from build123d import *

# Parameters (mm, degrees)
BOSS_EXTRUDE2_DEPTH = 39
SKETCH5_R           = 3
BOSS_EXTRUDE3_DEPTH = 0.75
BOSS_EXTRUDE5_DEPTH = 10
SKETCH10_R          = 2.25
BOSS_EXTRUDE6_DEPTH = 0.5


with BuildPart() as part:
    # Sketch4 → Boss-Extrude2 (new body)
    with BuildSketch(Plane(origin=(0, 0, 0), x_dir=(1, 0, 0), z_dir=(0, 1, 0))):
        with BuildLine():
            Line((-0.32, 1.337245303), (-0.32, 0.32))
            Line((-0.32, 0.32), (-1.337245303, 0.32))
            ThreePointArc((-1.337245303, 0.32), (-1.375, 0), (-1.337245303, -0.32))
            Line((-1.337245303, -0.32), (-0.32, -0.32))
            Line((-0.32, -0.32), (-0.32, -1.337245303))
            ThreePointArc((-0.32, -1.337245303), (0, -1.375), (0.32, -1.337245303))
            Line((0.32, -1.337245303), (0.32, -0.32))
            Line((0.32, -0.32), (1.337245303, -0.32))
            ThreePointArc((1.337245303, -0.32), (1.375, 0), (1.337245303, 0.32))
            Line((1.337245303, 0.32), (0.32, 0.32))
            Line((0.32, 0.32), (0.32, 1.337245303))
            ThreePointArc((0.32, 1.337245303), (0, 1.375), (-0.32, 1.337245303))
        make_face()
    extrude(amount=BOSS_EXTRUDE2_DEPTH)

    # Sketch5 → Boss-Extrude3 (add)
    with BuildSketch(Plane(origin=(0, 39, 0), x_dir=(1, 0, 0), z_dir=(0, 1, 0))):
        with Locations(Location((0, 0, 0), (0, 0, 270))):
            Circle(SKETCH5_R)
    extrude(amount=BOSS_EXTRUDE3_DEPTH)

    # Sketch9 → Boss-Extrude5 (add)
    with BuildSketch(Plane(origin=(0, 39.75, 0), x_dir=(1, 0, 0), z_dir=(0, 1, 0))):
        with BuildLine():
            Line((-0.83040283, -2.358056645), (-0.873204905, -2.479599724))
            ThreePointArc((-0.873204905, -2.479599724), (-0.653770741, -2.546268921), (-0.429360987, -2.593559473))
            Line((-0.429360987, -2.593559473), (-0.408314906, -2.466430404))
            ThreePointArc((-0.408314906, -2.466430404), (-0.313333084, -2.480286753), (-0.217889357, -2.490486745))
            Line((-0.217889357, -2.490486745), (-0.229120191, -2.618855769))
            ThreePointArc((-0.229120191, -2.618855769), (0, -2.628859372), (0.229120191, -2.618855769))
            Line((0.229120191, -2.618855769), (0.217889357, -2.490486745))
            ThreePointArc((0.217889357, -2.490486745), (0.313333084, -2.480286753), (0.408314906, -2.466430404))
            Line((0.408314906, -2.466430404), (0.429360987, -2.593559473))
            ThreePointArc((0.429360987, -2.593559473), (0.653770741, -2.546268921), (0.873204905, -2.479599724))
            Line((0.873204905, -2.479599724), (0.83040283, -2.358056645))
            ThreePointArc((0.83040283, -2.358056645), (0.920311382, -2.324441215), (1.008863241, -2.28739917))
            Line((1.008863241, -2.28739917), (1.060863834, -2.405300298))
            ThreePointArc((1.060863834, -2.405300298), (1.266462661, -2.303687029), (1.462422943, -2.18454131))
            Line((1.462422943, -2.18454131), (1.390739039, -2.077461173))
            ThreePointArc((1.390739039, -2.077461173), (1.469463131, -2.022542486), (1.546020988, -1.964642233))
            Line((1.546020988, -1.964642233), (1.625708706, -2.065907259))
            ThreePointArc((1.625708706, -2.065907259), (1.799578075, -1.916356008), (1.959751569, -1.752220131))
            Line((1.959751569, -1.752220131), (1.863689999, -1.666331176))
            ThreePointArc((1.863689999, -1.666331176), (1.926283107, -1.593559974), (1.986036551, -1.518439599))
            Line((1.986036551, -1.518439599), (2.088404321, -1.596705669))
            ThreePointArc((2.088404321, -1.596705669), (2.21961938, -1.408613292), (2.333941796, -1.209800517))
            Line((2.333941796, -1.209800517), (2.219538463, -1.150499462))
            ThreePointArc((2.219538463, -1.150499462), (2.262067631, -1.064448229), (2.301262134, -0.976827821))
            Line((2.301262134, -0.976827821), (2.419877811, -1.027177189))
            ThreePointArc((2.419877811, -1.027177189), (2.500193836, -0.812362222), (2.561481877, -0.591364688))
            Line((2.561481877, -0.591364688), (2.435925162, -0.562377636))
            ThreePointArc((2.435925162, -0.562377636), (2.455718127, -0.468453286), (2.471890953, -0.373838359))
            Line((2.471890953, -0.373838359), (2.599301479, -0.393107389))
            ThreePointArc((2.599301479, -0.393107389), (2.623671919, -0.165067446), (2.628074631, 0.064228761))
            Line((2.628074631, 0.064228761), (2.499253724, 0.061080445))
            ThreePointArc((2.499253724, 0.061080445), (2.495066821, 0.156976299), (2.487201772, 0.252640743))
            Line((2.487201772, 0.252640743), (2.615401476, 0.265662794))
            ThreePointArc((2.615401476, 0.265662794), (2.582295045, 0.492599125), (2.52953579, 0.715786479))
            Line((2.52953579, 0.715786479), (2.405544984, 0.680700618))
            ThreePointArc((2.405544984, 0.680700618), (2.377641291, 0.772542486), (2.346232557, 0.863245497))
            Line((2.346232557, 0.863245497), (2.467166179, 0.907740407))
            ThreePointArc((2.467166179, 0.907740407), (2.378663077, 1.119313881), (2.272056913, 1.322368701))
            Line((2.272056913, 1.322368701), (2.160687005, 1.257549867))
            ThreePointArc((2.160687005, 1.257549867), (2.110819814, 1.339566987), (2.057840921, 1.419609363))
            Line((2.057840921, 1.419609363), (2.163909757, 1.492781351))
            ThreePointArc((2.163909757, 1.492781351), (2.02557096, 1.67569803), (1.871816344, 1.845861634))
            Line((1.871816344, 1.845861634), (1.780065115, 1.755382632))
            ThreePointArc((1.780065115, 1.755382632), (1.711367765, 1.822421569), (1.640147572, 1.886773951))
            Line((1.640147572, 1.886773951), (1.724686927, 1.984025353))
            ThreePointArc((1.724686927, 1.984025353), (1.545204769, 2.126791908), (1.35396267, 2.253372292))
            Line((1.35396267, 2.253372292), (1.287595187, 2.142918252))
            ThreePointArc((1.287595187, 2.142918252), (1.204384185, 2.1907667), (1.11939772, 2.235385592))
            Line((1.11939772, 2.235385592), (1.177095675, 2.350605746))
            ThreePointArc((1.177095675, 2.350605746), (0.96774768, 2.444251629), (0.751034542, 2.519295281))
            Line((0.751034542, 2.519295281), (0.714220919, 2.395806436))
            ThreePointArc((0.714220919, 2.395806436), (0.621724718, 2.421457903), (0.528311991, 2.443539736))
            Line((0.528311991, 2.443539736), (0.555543172, 2.569488934))
            ThreePointArc((0.555543172, 2.569488934), (0.329483446, 2.608130031), (0.100916152, 2.626921683))
            Line((0.100916152, 2.626921683), (0.095969523, 2.498157291))
            ThreePointArc((0.095969523, 2.498157291), (0, 2.5), (-0.095969523, 2.498157291))
            Line((-0.095969523, 2.498157291), (-0.100916152, 2.626921683))
            ThreePointArc((-0.100916152, 2.626921683), (-0.329483446, 2.608130031), (-0.555543172, 2.569488934))
            Line((-0.555543172, 2.569488934), (-0.528311991, 2.443539736))
            ThreePointArc((-0.528311991, 2.443539736), (-0.621724718, 2.421457903), (-0.714220919, 2.395806436))
            Line((-0.714220919, 2.395806436), (-0.751034542, 2.519295281))
            ThreePointArc((-0.751034542, 2.519295281), (-0.96774768, 2.444251629), (-1.177095675, 2.350605746))
            Line((-1.177095675, 2.350605746), (-1.11939772, 2.235385592))
            ThreePointArc((-1.11939772, 2.235385592), (-1.204384185, 2.1907667), (-1.287595187, 2.142918252))
            Line((-1.287595187, 2.142918252), (-1.35396267, 2.253372292))
            ThreePointArc((-1.35396267, 2.253372292), (-1.545204769, 2.126791908), (-1.724686927, 1.984025353))
            Line((-1.724686927, 1.984025353), (-1.640147572, 1.886773951))
            ThreePointArc((-1.640147572, 1.886773951), (-1.711367765, 1.822421569), (-1.780065115, 1.755382632))
            Line((-1.780065115, 1.755382632), (-1.871816344, 1.845861634))
            ThreePointArc((-1.871816344, 1.845861634), (-2.02557096, 1.67569803), (-2.163909757, 1.492781351))
            Line((-2.163909757, 1.492781351), (-2.057840921, 1.419609363))
            ThreePointArc((-2.057840921, 1.419609363), (-2.110819814, 1.339566987), (-2.160687005, 1.257549867))
            Line((-2.160687005, 1.257549867), (-2.272056913, 1.322368701))
            ThreePointArc((-2.272056913, 1.322368701), (-2.378663077, 1.119313881), (-2.467166179, 0.907740407))
            Line((-2.467166179, 0.907740407), (-2.346232557, 0.863245497))
            ThreePointArc((-2.346232557, 0.863245497), (-2.377641291, 0.772542486), (-2.405544984, 0.680700618))
            Line((-2.405544984, 0.680700618), (-2.52953579, 0.715786479))
            ThreePointArc((-2.52953579, 0.715786479), (-2.582295045, 0.492599125), (-2.615401476, 0.265662794))
            Line((-2.615401476, 0.265662794), (-2.487201772, 0.252640743))
            ThreePointArc((-2.487201772, 0.252640743), (-2.495066821, 0.156976299), (-2.499253724, 0.061080445))
            Line((-2.499253724, 0.061080445), (-2.628074631, 0.064228761))
            ThreePointArc((-2.628074631, 0.064228761), (-2.623671919, -0.165067446), (-2.599301479, -0.393107389))
            Line((-2.599301479, -0.393107389), (-2.471890953, -0.373838359))
            ThreePointArc((-2.471890953, -0.373838359), (-2.455718127, -0.468453286), (-2.435925162, -0.562377636))
            Line((-2.435925162, -0.562377636), (-2.561481877, -0.591364688))
            ThreePointArc((-2.561481877, -0.591364688), (-2.500193836, -0.812362222), (-2.419877811, -1.027177189))
            Line((-2.419877811, -1.027177189), (-2.301262134, -0.976827821))
            ThreePointArc((-2.301262134, -0.976827821), (-2.262067631, -1.064448229), (-2.219538463, -1.150499462))
            Line((-2.219538463, -1.150499462), (-2.333941796, -1.209800517))
            ThreePointArc((-2.333941796, -1.209800517), (-2.21961938, -1.408613292), (-2.088404321, -1.596705669))
            Line((-2.088404321, -1.596705669), (-1.986036551, -1.518439599))
            ThreePointArc((-1.986036551, -1.518439599), (-1.926283107, -1.593559974), (-1.863689999, -1.666331176))
            Line((-1.863689999, -1.666331176), (-1.959751569, -1.752220131))
            ThreePointArc((-1.959751569, -1.752220131), (-1.799578075, -1.916356008), (-1.625708706, -2.065907259))
            Line((-1.625708706, -2.065907259), (-1.546020988, -1.964642233))
            ThreePointArc((-1.546020988, -1.964642233), (-1.469463131, -2.022542486), (-1.390739039, -2.077461173))
            Line((-1.390739039, -2.077461173), (-1.462422943, -2.18454131))
            ThreePointArc((-1.462422943, -2.18454131), (-1.266462661, -2.303687029), (-1.060863834, -2.405300298))
            Line((-1.060863834, -2.405300298), (-1.008863241, -2.28739917))
            ThreePointArc((-1.008863241, -2.28739917), (-0.920311382, -2.324441215), (-0.83040283, -2.358056645))
        make_face()
    extrude(amount=BOSS_EXTRUDE5_DEPTH)

    # Sketch10 → Boss-Extrude6 (add)
    with BuildSketch(Plane(origin=(0, 49.75, 0), x_dir=(1, 0, 0), z_dir=(0, 1, 0))):
        with Locations(Location((0, 0, 0), (0, 0, 270))):
            Circle(SKETCH10_R)
    extrude(amount=BOSS_EXTRUDE6_DEPTH)


solid = part.part
Can you work these out from the model? Positions are in its coordinate system, mm. A direction names the side the tool comes from. Give positions to 0.01 mm unless a question says otherwise; leave off trailing zeros. Loops run counter-clockwise (first coordinate to the right, second up) from the corner with the lowest first, then second, coordinate; pieces in that order, holes last. Notation, with made-up numbers: (32.25, 16) -> (46.25, 16) arc R25 ccw to (46.25, 34) -> close; hole circle Ø11 at (42, 60.25). An arc over 180 degrees is marked (long way). Write item = value, one per line.
1) For faces 1 (the flat face through (-0.32, 19, -1)), 2 (the flat face through (0.32, 19, -1)), 3 (the flat face through (1, 19, 0.32)), 4 (the flat face through (-0.32, 19, 1)), which set-ups out of +Z, -Z, +X, -X, +Y, -Y let a thin tool reach every point of the face, with its end or its side?
Check result:
face_1 = -Z, -X, -Y
face_2 = -Z, +X, -Y
face_3 = +Z, +X, -Y
face_4 = +Z, -X, -Y
2) Suppose I cut it at A-A on y = 5. Write out the boundary of the cut face in (x, z) (3 decimals).
Check result:
outline = (-1.337, -0.32) -> (-0.32, -0.32) -> (-0.32, -1.337) arc R1.375 ccw to (0.32, -1.337) -> (0.32, -0.32) -> (1.337, -0.32) arc R1.375 ccw to (1.337, 0.32) -> (0.32, 0.32) -> (0.32, 1.337) arc R1.375 ccw to (-0.32, 1.337) -> (-0.32, 0.32) -> (-1.337, 0.32) arc R1.375 ccw to start
3) I need wall thicknesses on L1, parallel to X at y = 24, z = -0.6; L2, parallel to Y at x = 0.35, z = 1.5. Which ranges of each line are inside material? Lowest first, please. Write a range as from..to.
Check result:
L1 = -0.32..0.32
L2 = 39..50.25
4) Will these pins go through, and if not, where does the flat tip stop? pin 1 (0.5 mm diameter, centred on x = -1, y = 10, fed in from -Z); pin 2 (1.1 mm diameter, centred on y = 13, z = 1, fed in from -X); pin 3 (0.5 mm diameter, centred on x = -1, y = 24, fed in from +Z); pin 4 (1.5 mm diameter, centred on x = 1, z = 0.5, fed in from -Y).
Check result:
pin_1 = -0.32
pin_2 = -0.32
pin_3 = 0.32
pin_4 = 0
